Model file for the job. Use its own axes, mm. A direction names the side the tool comes from. Coordinates: 2 decimals unless noted, no trailing zeros. Order: outer loops, then holes, each group sorted by start corner. A loop starts at its lowest first (then second) coordinate and runs counter-clockwise, first axis right, second up. Notation, with made-up numbers: (-9, 19.5) -> (-3, 19.5) arc R27 cw to (-3, 53.5) -> close; hole circle Ø4 at (31.25, 41). An arc over 180 degrees is marked (long way). Return JSON: item names as keys, results as strings. Group by question number.
1) Cut at A-A (z = 0). Write the cut outline in (x, y), and give its area (3 significant figures).
2) Flat gauge pins, fed straight in: pin 1 (12 mm diameter, centred on x = 12.5, z = 5, fed in from +Y); pin 2 (2 mm diameter, centred on x = 36, y = 0.5, fed in from +Z); pin 3 (1.5 mm diameter, centred on y = -7.5, z = 3, fed in from +X). Where does each tip first touch, or does it go through?
3) Cut at D-D (x = 37). Write the cut outline in (y, z), and give its area (3 significant figures).
4) Which spindle directions (+Z, -Z, +X, -X, +Y, -Y) get a long thin tool onto all of the face, cutting with end or side? Do faces 5 (the cylindrical face through (2.3, -1.6, 5)), 6 (the flat face through (43.62, -0.61, 0.03)), 7 (the flat face through (28, 3, -2)), 8 (the flat face through (39.6, -5.39, 0.03)). Say none if no direction does.
5) Cut at C-C (x = 13). Write the cut outline in (y, z), and give its area (3 significant figures).
6) Probe line 1 (Z direction, x = 35, y = 7.5); line 2 (Y direction, x = 2.35, z = 0); line 3 (Z direction, x = 7.5, y = 1.25). List the from-to ranges inside material, lowest first.
7) Cut at B-B (x = 4). Write the cut outline in (y, z).
8) Pull direction Z, two halves, no side cores. Call faces 1 (the flat face through (28, 3, 2)), 2 (the flat face through (1, 0, 0)), 3 (the flat face through (0, 0, 0)), 4 (the flat face through (3.5, 0, 0)): +Z half, -Z half, draft (parallel to the pull), parting line (faces both ways), or undercut.
from build123d import *

# Parameters (mm, degrees)
EXTRUDE_2037_DEPTH = 2


with BuildPart() as part:
    # Sketch 227 → Повернуть1 (revolve)
    with BuildSketch(Plane.XY, mode=Mode.PRIVATE) as revolve_1_sk:
        with BuildLine():
            Line((0, 10.929858877), (0, 0))
            Line((0, 0), (1, 0))
            Line((1, 0), (1, 5.25))
            Line((1, 5.25), (3.5, 5.25))
            Line((3.5, 5.25), (3.5, 0))
            Line((3.5, 0), (8, 0))
            Line((8, 0), (8, 8))
            ThreePointArc((8, 8), (7.096901825, 10.076121155), (5, 10.929858877))
            Line((5, 10.929858877), (0, 10.929858877))
        make_face()
        with BuildLine():
            ThreePointArc((11.2, 4.8), (10.2627417, 7.0627417), (8, 8))
            Line((8, 8), (8, 0))
            Line((8, 0), (11.2, 0))
            Line((11.2, 0), (11.2, 2.4))
            Line((11.2, 2.4), (11.2, 4.8))
        make_face()
    revolve(revolve_1_sk.sketch.rotate(Axis((0, 0, 0), (1, 0, 0)), 90), axis=Axis((0, 0, 0), (1, 0, 0)))

    # Sketch 1020 → Extrude 2037 (add, symmetric)
    with BuildSketch(Plane.XY):
        with BuildLine():
            ThreePointArc((11.2, 4.4), (29.338267199, 10.995701086), (45.2, 0))
            Line((45.2, 0), (11.2, 0))
            Line((11.2, 0), (11.2, 4.4))
        make_face()
        with BuildLine():
            Line((31.263463773, 0), (11.2, 0))
            Line((11.2, 0), (11.2, -3.914978255))
            ThreePointArc((11.2, -3.914978255), (22.080678837, -6.30816882), (31.263463773, 0))
        make_face()
        Polygon((38.912013935, 0), (35.248695767, 0), (35.248695767, -11.07), (38.912013935, -4.32), align=None)
        Polygon((35.248695767, 0), (31.263463773, 0), (32.498964702, -1.197255299), (32.498964702, -9.797255299), (35.248695767, -11.07), align=None)
        Polygon((42.083014277, -1.2), (42.083014277, 0), (40.307542508, 0), (40.307542508, -6.49), align=None)
        Polygon((40.307542508, 0), (38.912013935, 0), (38.912013935, -4.32), (40.307542508, -6.49), align=None)
        Polygon((42.083014277, -1.2), (45.2, 0), (42.083014277, 0), align=None)
    extrude(amount=EXTRUDE_2037_DEPTH, both=True)


solid = part.part
Answers below:
{
 "1": {"outline": "(0, -10.93) -> (5, -10.93) arc R3 ccw to (8, -8) arc R3.2 ccw to (11.2, -4.8) -> (11.2, -3.91) arc R14 ccw to (31.26, 0) -> (32.5, -1.2) -> (32.5, -9.8) -> (35.25, -11.07) -> (38.91, -4.32) -> (40.31, -6.49) -> (42.08, -1.2) -> (45.2, 0) arc R21 ccw to (11.2, 4.4) -> (11.2, 4.8) arc R3.2 ccw to (8, 8) arc R3 ccw to (5, 10.93) -> (0, 10.93) -> close; hole (1, -5.25) -> (3.5, -5.25) -> (3.5, 5.25) -> (1, 5.25) -> close", "area": "655 mm^2"},
 "2": {"pin 1": "stops at y = 9.85", "pin 2": "stops at z = 2", "pin 3": "stops at x = 9.96"},
 "3": {"outline": "(-7.84, -2) -> (8.44, -2) -> (8.44, 2) -> (-7.84, 2) -> close", "area": "65.1 mm^2"},
 "4": {"face 5": "none", "face 6": "+Z, -Z, +X, -Y", "face 7": "-Z, +X, +Y, -Y", "face 8": "+Z, -Z, -Y"},
 "5": {"outline": "(-5.02, -2) -> (6.13, -2) -> (6.13, 2) -> (-5.02, 2) -> close", "area": "44.6 mm^2"},
 "6": {"line 1": "z = -2 to 2", "line 2": "y = -10.93 to -5.25, 5.25 to 10.93", "line 3": "z = -9.51 to 9.51"},
 "7": {"outline": "circle Ø21.86 at (0, 0)"},
 "8": {"face 1": "+Z half", "face 2": "undercut", "face 3": "draft", "face 4": "undercut"}
}
